Here's the drawing with two shaded views (mm, measured from the low corner). I have some questions. A direction names the side the tool comes from. Round coordinates to 2 decimals unless told otherwise and drop trailing zeros. Order: outer loops, then holes, each group sorted by start corner. A loop starts at its lowest first (then second) coordinate and runs counter-clockwise, first axis right, second up. Notation, with made-up numbers: (47, 77.25) - (100, 77.25) arc R24 ccw to (100, 110.25) - close; hole circle Ø2 at (87.25, -19.5). An arc over 180 degrees is marked (long way). One line per item, written item: value.
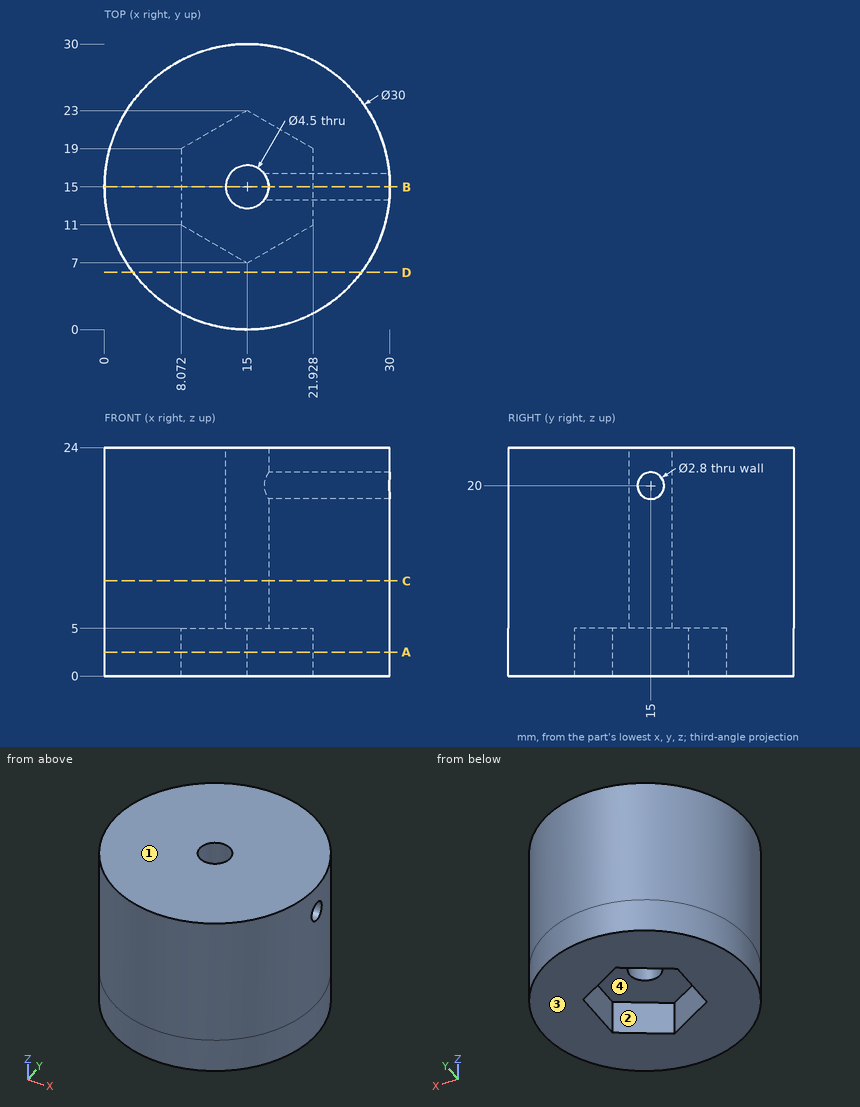
Q1. Will these pins go through, and if not, where does the flat tip stop? pin 1 (2.5 mm diameter, centred on y = 13, z = 3, fed in from +X); pin 2 (12 mm diameter, centred on x = 24, z = 4, fed in from -Y); pin 3 (8 mm diameter, centred on y = 23.5, z = 16.5, fed in from -X).
Results list:
pin 1: x = 29.98
pin 2: y = 0.3
pin 3: x = 0.69
Q2. If we section it at D-D, the plane y = 6: Please give me the cut outline in (x, z), then the cut area to 3 significant figures.
Results list:
outline: (3, 0) - (27, 0) - (27, 24) - (3, 24) - close
area: 576 mm²
Q3. If we section it at A-A, the plane z = 2.5: Please give me the cut outline in (x, y).
Results list:
outline: circle Ø30 at (15, 15); hole (8.07, 11) - (15, 7) - (21.93, 11) - (21.93, 19) - (15, 23) - (8.07, 19) - close
Q4. We'd pull the mould along X, two halves only. Please class the marked faces 3 and 4: released by +X, released by -X, zero draft, split by the parting line, or undercut.
Results list:
face 3: zero draft
face 4: undercut
Q5. If we section it at B-B, the plane y = 15: Please give me the cut outline in (x, z).
Results list:
outline: (0, 0) - (8.07, 0) - (8.07, 5) - (12.75, 5) - (12.75, 24) - (0, 24) - close; (17.25, 5) - (21.93, 5) - (21.93, 0) - (30, 0) - (30, 18.6) - (17.25, 18.6) - close; (17.25, 21.4) - (30, 21.4) - (30, 24) - (17.25, 24) - close
Q6. If I drill on line 1 along Y through (x, z) = (15, 13.5); line 2 along Z through (x, y) = (10, 16.5); line 3 along X through (y, z) = (22, 1.75) (1 decimal), over which ranges is the centre line in solid material (lowest first)?
Results list:
line 1: 0 to 12.75, 17.25 to 30
line 2: 5 to 24
line 3: 1.7 to 13.3, 16.7 to 28.3
Q7. Which directions (+Z, -Z, +X, -X, +Y, -Y) give clear straight access to the entire face, cutting with the end or side of a thin tool? Please do the marked faces 1 and 2.
Results list:
face 1: +Z, +X, -X, +Y, -Y
face 2: -Z
Q8. If we section it at C-C, the plane z = 10: Please give me the cut outline in (x, y).
Results list:
outline: circle Ø30 at (15, 15); hole circle Ø4.5 at (15, 15)
